Part model, mm, in its own coordinate system. A direction names the side the tool comes from. Coordinates: 2 decimals unless noted, no trailing zeros. Order: outer loops, then holes, each group sorted by start corner. A loop starts at its lowest first (then second) coordinate and runs counter-clockwise, first axis right, second up.
1) Tool access for faces 5 (the flat face through (2, 3, 10)), 6 (the flat face through (88, 30, 45)), 7 (the flat face through (45, 30, 20)): list every direction of +Z, -Z, +X, -X, +Y, -Y with a clear straight run to the whole face (end or side of a thin tool).
2) Wall check: L1, parallel to Y at x = 30, z = 13; L2, parallel to Z at x = 18, y = 11; L3, parallel to X at y = 6.5, z = 26.5. Give the ranges that are in metal, low to high.
3) Cut at B-B (y = 30). List the corners of the cut face in (x, z), and give its area (3 significant figures).
4) Cut at A-A (x = 78). List the corners of the cut face in (y, z).
5) Pin check, flat tips, straight feed: pin 1 Ø10 at (x, y) = (24, 9.5) entering from -Z; pin 2 Ø3 at (x, y) = (60, 22.5) entering from +Z; pin 3 Ø10 at (y, z) = (9.5, 45) entering from -X. Stop position of each tip, or through.
6) Cut at C-C (z = 16.5). List the corners of the cut face in (x, y), and give its area (3 significant figures).
7) Cut at D-D (x = 30.5). List the corners of the cut face in (y, z), and give its area (3 significant figures).
8) Mould opens along Z. For faces 1 (the flat face through (49, 30, 0)), 2 (the flat face through (59, 60, 14)), 3 (the flat face through (88, 30, 35)), 4 (the cylindrical face through (87.7, 12.5, 40.1)) say: +Z half, -Z half, draft (parallel to the pull), parting line (faces both ways), or undercut.
```python
from build123d import *

# Parameters (mm, degrees)
SKETCH_W     = 100
SKETCH_H     = 60
SKETCH_R     = 12.5
PAD_DEPTH    = 20
SKETCH001_W  = 25
SKETCH001_H  = 60
PAD001_DEPTH = 30
POCKET_DEPTH = 25
FILLET_R     = 5
CHAMFER_SIZE = 5


with BuildPart() as part:
    # Sketch → Pad (new body)
    with BuildSketch(Plane.XY):
        with Locations((50, 30)):
            Rectangle(SKETCH_W, SKETCH_H)
        with Locations((30, 30)):
            Circle(SKETCH_R, mode=Mode.SUBTRACT)
    extrude(amount=PAD_DEPTH)

    # Sketch001 (on Face7 of Pad) → Pad001 (join)
    with BuildSketch(Plane.XY.offset(20)):
        with Locations((87.5, 30)):
            Rectangle(SKETCH001_W, SKETCH001_H)
    extrude(amount=PAD001_DEPTH)

    # Sketch002 (on Face8 of Pad001) → Pocket (cut)
    with BuildSketch(Plane.YZ.offset(100)):
        with BuildLine():
            ThreePointArc((17.5, 45), (12.5, 40), (17.5, 35))
            Line((17.5, 35), (42.5, 35))
            ThreePointArc((42.5, 35), (47.5, 40), (42.5, 45))
            Line((42.5, 45), (17.5, 45))
        make_face()
    extrude(amount=-POCKET_DEPTH, mode=Mode.SUBTRACT)

    # Fillet
    fillet_edges = [part.edges().sort_by_distance(p)[0] for p in [
        (100, 0, 25),
        (100, 60, 25),
    ]]
    fillet(fillet_edges, radius=FILLET_R)

    # Chamfer
    chamfer_edges = [part.edges().sort_by_distance(p)[0] for p in [
        (0, 0, 10),
        (0, 60, 10),
    ]]
    chamfer(chamfer_edges, length=CHAMFER_SIZE)


solid = part.part
```
Geometry check:
1. face 5: +Z, -Z, -X, -Y
1. face 6: +X, -X
1. face 7: +Z, -X, +Y, -Y
2. L1: y = 0 to 17.5, 42.5 to 60
2. L2: z = 0 to 20
2. L3: x = 75 to 100
3. outline: (0, 0) - (17.5, 0) - (17.5, 20) - (0, 20) - close; (42.5, 0) - (100, 0) - (100, 35) - (75, 35) - (75, 20) - (42.5, 20) - close; (75, 45) - (100, 45) - (100, 50) - (75, 50) - close
3. area: 2,000 mm2
4. outline: (0, 0) - (60, 0) - (60, 50) - (0, 50) - close; hole (17.5, 35) - (42.5, 35) arc R5 ccw to (42.5, 45) - (17.5, 45) arc R5 ccw to start
5. pin 1: stops at z = 0
5. pin 2: stops at z = 20
5. pin 3: stops at x = 75
6. outline: (0, 5) - (5, 0) - (95, 0) arc R5 ccw to (100, 5) - (100, 55) arc R5 ccw to (95, 60) - (5, 60) - (0, 55) - close; hole circle Ø25 at (30, 30)
6. area: 5,470 mm2
7. outline: (0, 0) - (17.51, 0) - (17.51, 20) - (0, 20) - close; (42.49, 0) - (60, 0) - (60, 20) - (42.49, 20) - close
7. area: 700 mm2
8. face 1: -Z half
8. face 2: draft
8. face 3: undercut
8. face 4: undercut
